Print and shaded views of the part. All mm, measured from the part's lowest x, y and z. Round coordinates to 2 decimals unless told otherwise and drop trailing zeros. Loops run counter-clockwise (first coordinate to the right, second up) from the corner with the lowest first, then second, coordinate; pieces in that order, holes last. Notation, with made-up numbers: (-24, 45.25) - (-13, 45.25) arc R11 cw to (-13, 56.25) - close; hole circle Ø1 at (-30.75, -30). An arc over 180 degrees is marked (long way). Use one line per item in the form item = value. Start each with the question number.
Q1. Saw through at A-A (x = 94.38). Give the cut face in (y, z), then the cut area to 3 significant figures.
Q2. Pin check, flat tip, straight feed: pin 1 (1 mm diameter, centred on x = 22.5, y = 63.5, fed in from -Z). Stop position of the tip, or through.
Q3. Drill centre line: line 1 (Y direction, x = 8.03, z = 0.45). Where is it in solid material? Low to high.
Q4. Saw through at B-B (z = 0.95). Give the cut face in (x, y), then the cut area to 3 significant figures.
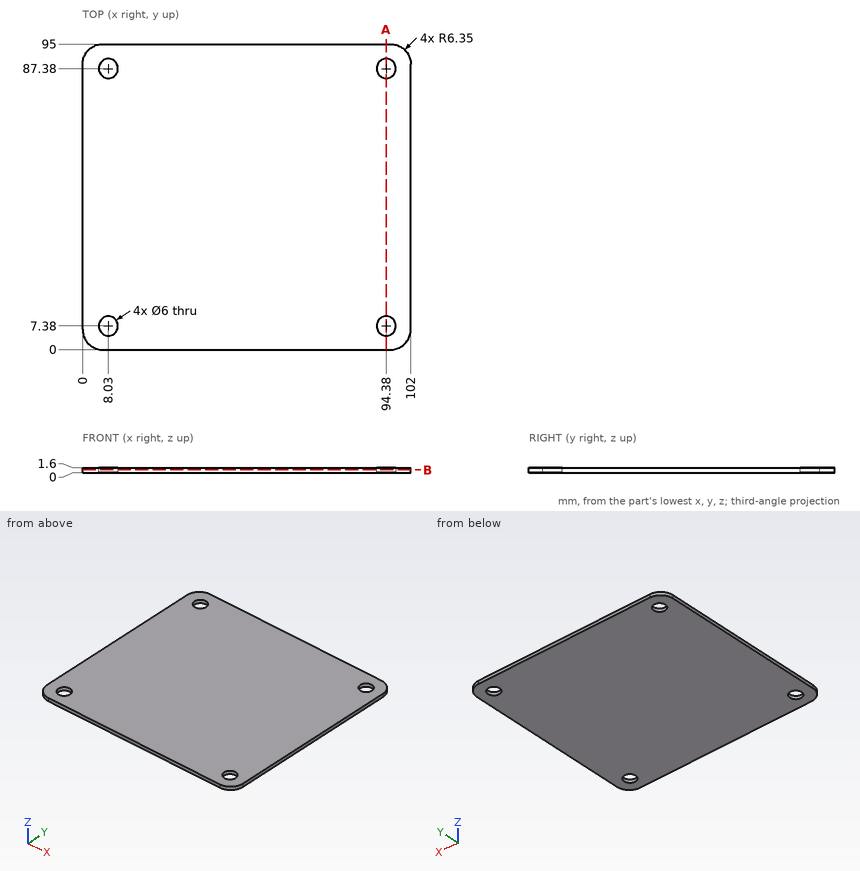
Report:
q1.outline = (0, 0) - (4.38, 0) - (4.38, 1.6) - (0, 1.6) - close; (10.38, 0) - (84.38, 0) - (84.38, 1.6) - (10.38, 1.6) - close; (90.38, 0) - (95, 0) - (95, 1.6) - (90.38, 1.6) - close
q1.area = 133 mm²
q2.pin_1 = 0
q3.line_1 = 0 to 4.38, 10.38 to 84.38, 90.38 to 95
q4.outline = (0, 6.35) arc R6.35 ccw to (6.35, 0) - (95.65, 0) arc R6.35 ccw to (102, 6.35) - (102, 88.65) arc R6.35 ccw to (95.65, 95) - (6.35, 95) arc R6.35 ccw to (0, 88.65) - close; hole circle Ø6 at (8.03, 7.38); hole circle Ø6 at (8.03, 87.38); hole circle Ø6 at (94.38, 7.38); hole circle Ø6 at (94.38, 87.38)
q4.area = 9,540 mm²
